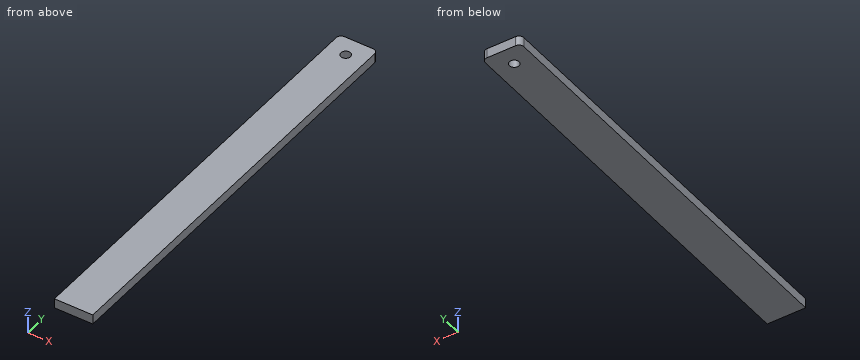
Solid Edge part; units mm, degrees
sketch "Sketch1" plane through (0, 0, 0) normal (0, 0, 1) x (1, 0, 0)
  line L0 (-12.7, -139.7) -> (12.7, -139.7)
  line L1 (12.7, -139.7) -> (12.7, 139.7)
  line L2 (12.7, 139.7) -> (-12.7, 139.7)
  line L3 (-12.7, 139.7) -> (-12.7, -139.7)
  dimension "D1" = 12.7
  dimension "D2" = 12.7
extrude "Protrusion1" add sketch "Sketch1" along normal blind 6.35
hole "Hole_1" at (0, 127, 6.35) direction (0, 0, -1) diameter 6.35 end up to next
fillet "Round_1" radius 3.175 2 edges at (12.7, 139.7, 3.175) (-12.7, 139.7, 3.175)
properties part number "SPaRC - 02 - 002"
Here's how the part is built. I have some questions about the finished solid (model axes, mm). Round coordinates to 2 decimals unless told otherwise and drop trailing zeros. Write each loop counter-clockwise with the first axis right and the second up, starting at its lowest first coordinate (ties: lowest second). Pieces come first, ordered by that corner, then holes.
Q1. If we section it at A-A on x = 0: Write out the boundary of the cut face in (y, z) (3 decimals), plus the area to 3 significant figures.
Q2. Will this pin go through, and if not, where does the flat tip stop? P1, Ø5.5, axis at x = 0, y = 127, coming from the +Z side.
Q3. If we section it at B-B on y = 127: Write out the boundary of the cut face in (x, z) (3 decimals).
Q4. Please list where these lines run through material, in increasing order: probe 1 along Y at (x, z) = (0, 4.25) (3 decimals); probe 2 along Y at (x, z) = (-0.5, 3); probe 3 along X at (y, z) = (127, 5) (3 decimals).
Answer below:
1. outline: (-139.7, 0) - (123.825, 0) - (123.825, 6.35) - (-139.7, 6.35) - close; (130.175, 0) - (139.7, 0) - (139.7, 6.35) - (130.175, 6.35) - close
1. area: 1,730 mm2
2. P1: passes through
3. outline: (-12.7, 0) - (-3.175, 0) - (-3.175, 6.35) - (-12.7, 6.35) - close; (3.175, 0) - (12.7, 0) - (12.7, 6.35) - (3.175, 6.35) - close
4. probe 1: y = -139.7 to 123.825, 130.175 to 139.7
4. probe 2: y = -139.7 to 123.86, 130.14 to 139.7
4. probe 3: x = -12.7 to -3.175, 3.175 to 12.7
